Part model, mm, in its own coordinate system. Round coordinates to 2 decimals unless told otherwise and drop trailing zeros. Order: outer loops, then holes, each group sorted by start corner. A loop starts at its lowest first (then second) coordinate and runs counter-clockwise, first axis right, second up. Notation, with made-up numbers: M 55.5,4.5 L 107.5,4.5 A12 cw 107.5,8.5 Z; hole C 63.25,83.25 d7. An arc over 180 degrees is marked long. Write each question's results on one line, items separated by ' | '. Start each with the question number.
1. Band-saw the part on A-A, the plane x = 127. List the corners of the cut face in (y, z) (3 decimals).
2. Probe L1, parallel to Y at x = -127, z = 1.4; L2, parallel to X at y = 162, z = 0.6; L3, parallel to Y at x = 44.45, z = 0.75. List the from-to ranges inside material, lowest first. Write a range as [from, to].
3. Drop a flat-ended pin along its axis: pin 1 Ø15.5 at (x, y) = (127, 162.72) entering from +Z (3 decimals). Give the stop position or say it passes through.
4. Two-plate mould, pull along X, no slides. Class faces 1 (the face through (-2, 2, 3.175)), 2 (the face through (120.768, -165.303, 1.565)): +X half, -X half, draft (parallel to the pull), parting line (faces both ways), or undercut.
5. Band-saw the part on B-B, the plane z = 2.2. Give the number of separate pieces and of enclosed holes in the cut face, then the cut area to 3 significant figures.
```python
from build123d import *

# Parameters (mm, degrees)
SKETCH1_W                        = 304.8
SKETCH1_H                        = 355.6
BOSS_EXTRUDE1_DEPTH              = 3.175
F_17_32_0_53125_DIAMETER_HOLE1_D = 13.49375
FILLET1_R                        = 6.35
F_1_4_CLEARANCE_HOLE1_D          = 7.14248
SKETCH2_W                        = 31.75
SKETCH2_H                        = 25.4
CUT_EXTRUDE1_DEPTH               = 4.175
FILLET2_R                        = 1.5875


with BuildPart() as part:
    # Sketch1 → Boss-Extrude1 (new body)
    with BuildSketch(Plane.XY):
        Rectangle(SKETCH1_W, SKETCH1_H)
    extrude(amount=BOSS_EXTRUDE1_DEPTH)

    # 17/32 (0.53125) Diameter Hole1 (through all)
    with Locations(Plane.XY.offset(3.175)):
        with Locations((-127, 162.71875), (-127, 91.28125), (-127, -91.28125), (-127, -162.71875), (127, -162.71875), (127, -91.28125), (127, 91.28125), (127, 162.71875)):
            Hole(F_17_32_0_53125_DIAMETER_HOLE1_D / 2)

    # Fillet1
    fillet1_edges = [part.edges().sort_by_distance(p)[0] for p in [
        (152.4, -177.8, 1.5875),
        (-152.4, -177.8, 1.5875),
        (-152.4, 177.8, 1.5875),
        (152.4, 177.8, 1.5875),
    ]]
    fillet(fillet1_edges, radius=FILLET1_R)

    # 1/4 Clearance Hole1 (through all)
    with Locations(Plane(origin=(0, 0, 0), x_dir=(-1, 0, 0), z_dir=(0, 0, -1))):
        with Locations((-44.45, 56.9515625), (-44.45, -56.9515625), (44.45, 56.9515625), (44.45, -56.9515625)):
            Hole(F_1_4_CLEARANCE_HOLE1_D / 2)

    # Sketch2 → Cut-Extrude1 (cut, through all)
    with BuildSketch(Plane.XY.offset(3.175)):
        with Locations((0, -114.3)):
            Rectangle(SKETCH2_W, SKETCH2_H)
    extrude(amount=-CUT_EXTRUDE1_DEPTH, mode=Mode.SUBTRACT)

    # Fillet2
    fillet2_edges = [part.edges().sort_by_distance(p)[0] for p in [
        (-15.875, -101.6, 1.5875),
        (15.875, -101.6, 1.5875),
        (15.875, -127, 1.5875),
        (-15.875, -127, 1.5875),
    ]]
    fillet(fillet2_edges, radius=FILLET2_R)


solid = part.part
```
Solution:
1) outline: M -177.8,0 L -169.466,0 L -169.466,3.175 L -177.8,3.175 Z; M -155.972,0 L -98.028,0 L -98.028,3.175 L -155.972,3.175 Z; M -84.534,0 L 84.534,0 L 84.534,3.175 L -84.534,3.175 Z; M 98.028,0 L 155.972,0 L 155.972,3.175 L 98.028,3.175 Z; M 169.466,0 L 177.8,0 L 177.8,3.175 L 169.466,3.175 Z
2) L1: [-177.8, -169.47], [-155.97, -98.03], [-84.53, 84.53], [98.03, 155.97], [169.47, 177.8] | L2: [-152.4, -133.71], [-120.29, 120.29], [133.71, 152.4] | L3: [-177.8, -60.52], [-53.38, 53.38], [60.52, 177.8]
3) pin 1: z = 3.175
4) face 1: draft | face 2: undercut
5) separate pieces: 1 | enclosed holes: 13 | area: 106,000 mm^2
